Source: CAD feature listing. Evaluate the final solid. Frame: model axes, mm. Face numbers are marked on the shaded views. A direction names the side the tool comes from. Round coordinates to 2 decimals unless told otherwise and drop trailing zeros. Loops run counter-clockwise (first coordinate to the right, second up) from the corner with the lowest first, then second, coordinate; pieces in that order, holes last.
Item 1: First-contact query: P1, Ø7, axis at x = 0, z = 0, coming from the +Y side; P2, Ø14, axis at x = 70, z = 4.5, coming from the +Y side; P3, Ø3, axis at y = 10.5, z = -9, coming from the -X side. Flat tips, straight axial feed; report the tip coordinate or a pass-through.
Item 2: Section query A-A on y = 49.5. Return loops of the section in (x, z).
Item 3: Pull-direction query (X, two-part tool) for the marked faces 3, 4, 5 and 6; classes: released by +X, released by -X, zero draft, split by the parting line, or undercut.
Item 4: Section query C-C on z = 0. Give the number of separate pieces and of enclosed holes in the cut face, then the cut area to 3 significant figures.
Item 5: Ray query, L1, parallel to X at y = 42.5, z = 3; L2, parallel to X at y = 22, z = -2; L3, parallel to Y at x = -63.5, z = -7.5. Return the intervals inside material, ascending.
Item 6: Section query D-D on x = 0. Return loops of the section in (y, z).
Item 7: Access query for the marked faces 1 and 2. Directions: +Z, -Z, +X, -X, +Y, -Y. A direction counts if a zero-diameter tool reaches every point of the face in a straight line with its end or side. Return the directions, or none.
Item 8: Section query B-B on x = -65. Return loops of the section in (y, z), then the cut area to 3 significant figures.
```python
from build123d import *

# Parameters (mm, degrees)
BOSS_EXTRUDE1_DEPTH = 18
CUT_EXTRUDE1_DEPTH  = 43
SKETCH12_W          = 20
SKETCH12_H          = 20
CUT_EXTRUDE2_DEPTH  = 8
SKETCH13_R          = 4.5
CUT_EXTRUDE3_DEPTH  = 55
CUT_EXTRUDE4_DEPTH  = 12
CUT_EXTRUDE8_START  = -6
SKETCH18_R          = 3
CUT_EXTRUDE8_DEPTH  = 6.238337
FILLET1_R           = 6


with BuildPart() as part:
    # Sketch1 → Boss-Extrude1 (new body, symmetric)
    with BuildSketch(Plane.XY):
        with BuildLine():
            Line((82, 0), (-82, 0))
            Line((-82, 0), (-79, 11))
            Line((-79, 11), (-49, 11))
            Line((-49, 11), (-49, 54))
            Line((-49, 54), (-22, 54))
            Line((-22, 54), (-22, 41))
            Line((-22, 41), (-19, 41))
            Line((-19, 41), (-19, 38))
            ThreePointArc((-19, 38), (0, 19), (19, 38))
            Line((19, 38), (19, 41))
            Line((19, 41), (22, 41))
            Line((22, 41), (22, 54))
            Line((22, 54), (49, 54))
            Line((49, 54), (49, 11))
            Line((49, 11), (79, 11))
            Line((79, 11), (82, 0))
        make_face()
    extrude(amount=BOSS_EXTRUDE1_DEPTH, both=True)

    # Sketch3 → Cut-Extrude1 (cut)
    with BuildSketch(Plane(origin=(0, 54, 0), x_dir=(1, 0, 0), z_dir=(0, 1, 0))):
        with BuildLine():
            Line((-44.497190923, 18), (-49, 18))
            Line((-49, 18), (-49, -18))
            Line((-49, -18), (-44.497190923, -18))
            ThreePointArc((-44.497190923, -18), (-48, 0), (-44.497190923, 18))
        make_face()
        with BuildLine():
            Line((49, -18), (49, 18))
            Line((49, 18), (44.497190923, 18))
            ThreePointArc((44.497190923, 18), (48, 0), (44.497190923, -18))
            Line((44.497190923, -18), (49, -18))
        make_face()
    extrude(amount=-CUT_EXTRUDE1_DEPTH, mode=Mode.SUBTRACT)

    # Sketch12 → Cut-Extrude2 (cut)
    with BuildSketch(Plane.XZ):
        with Locations((-31, 0)):
            Rectangle(SKETCH12_W, SKETCH12_H)
        with Locations((31, 0)):
            Rectangle(SKETCH12_W, SKETCH12_H)
    extrude(amount=-CUT_EXTRUDE2_DEPTH, mode=Mode.SUBTRACT)

    # Sketch13 → Cut-Extrude3 (cut, through all)
    with BuildSketch(Plane(origin=(0, 54, 0), x_dir=(1, 0, 0), z_dir=(0, 1, 0))):
        with Locations(Location((-31, 0, 0), (0, 0, 270))):  # turned: the seam where the file's is
            Circle(SKETCH13_R)
        with Locations(Location((31, 0, 0), (0, 0, 270))):  # turned: the seam where the file's is
            Circle(SKETCH13_R)
    extrude(amount=-CUT_EXTRUDE3_DEPTH, mode=Mode.SUBTRACT)

    # Sketch14 → Cut-Extrude4 (cut, through all)
    with BuildSketch(Plane(origin=(0, 11, 0), x_dir=(1, 0, 0), z_dir=(0, 1, 0))):
        with BuildLine():
            Line((-67.5, 4.5), (-60.5, 4.5))
            ThreePointArc((-60.5, 4.5), (-56, 0), (-60.5, -4.5))
            Line((-60.5, -4.5), (-67.5, -4.5))
            ThreePointArc((-67.5, -4.5), (-72, 0), (-67.5, 4.5))
        make_face()
        with BuildLine():
            Line((67.5, 4.5), (60.5, 4.5))
            ThreePointArc((60.5, 4.5), (56, 0), (60.5, -4.5))
            Line((60.5, -4.5), (67.5, -4.5))
            ThreePointArc((67.5, -4.5), (72, 0), (67.5, 4.5))
        make_face()
    extrude(amount=-CUT_EXTRUDE4_DEPTH, mode=Mode.SUBTRACT)

    # Sketch18 → Cut-Extrude8 (cut)
    with BuildSketch(Plane(origin=(0, 19, 0), x_dir=(1, 0, 0), z_dir=(0, 1, 0)).offset(CUT_EXTRUDE8_START)):
        with Locations(Location((0, 0, 0), (0, 0, 270))):  # turned: the seam where the file's is
            Circle(SKETCH18_R)
    extrude(amount=CUT_EXTRUDE8_DEPTH, mode=Mode.SUBTRACT)

    # Fillet1
    fillet1_edges = [part.edges().sort_by_distance(p)[0] for p in [
        (-48, 11, 0),
        (48, 11, 0),
    ]]
    fillet(fillet1_edges, radius=FILLET1_R)


solid = part.part
```
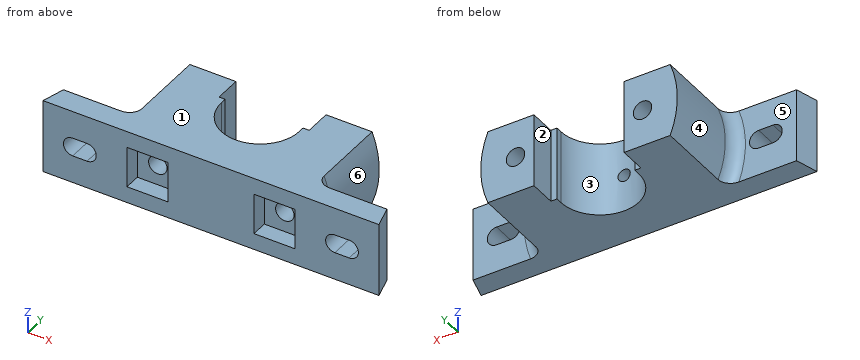
Data:
1. P1: stops at y = 19.33
1. P2: stops at y = 11
1. P3: stops at x = -79.55
2. outline: (-44.5, -18) - (-22, -18) - (-22, 18) - (-44.5, 18) arc R48 ccw to start; (22, -18) - (44.5, -18) arc R48 ccw to (44.5, 18) - (22, 18) - close; hole circle Ø9 at (-31, 0); hole circle Ø9 at (31, 0)
3. face 3: undercut
3. face 4: released by -X
3. face 5: zero draft
3. face 6: released by +X
4. separate pieces: 5
4. enclosed holes: 0
4. area: 3,120 mm2
5. L1: x = -47.91 to -34.35, -27.65 to -22, 22 to 27.65, 34.35 to 47.91
5. L2: x = -47.96 to -35.03, -26.97 to -10.25, 10.25 to 26.97, 35.03 to 47.96
5. L3: y = 0 to 11
6. outline: (0, -18) - (19, -18) - (19, -3) - (13, -3) - (13, 3) - (19, 3) - (19, 18) - (0, 18) - close
7. face 1: +Z, +X, -X, +Y, -Y
7. face 2: +Z, -Z, +Y
8. outline: (0, -18) - (11, -18) - (11, -4.5) - (0, -4.5) - close; (0, 4.5) - (11, 4.5) - (11, 18) - (0, 18) - close
8. area: 297 mm2
